Check sheet for the modelled part. Datum: model origin and axes. Units: mm. Face numbers are marked on the shaded views. A direction names the side the tool comes from. Give positions to 0.01 mm unless a question says otherwise; leave off trailing zeros. Order: outer loops, then holes, each group sorted by start corner. A loop starts at its lowest first (then second) coordinate and runs counter-clockwise, first axis right, second up. Notation, with made-up numbers: (61, 49) -> (119, 49) arc R18 cw to (119, 75) -> close; hole circle Ø5 at (-4.5, 14). An arc over 180 degrees is marked (long way). Write each question's results on one line, items separated by ' | '.
from build123d import *

# Parameters (mm, degrees)
F0_W     = 60
F0_H     = 30
F1_DEPTH = 5
F2_R     = 2.5
F3_DEPTH = 20
F4_R     = 0.75
F5_DEPTH = 23


with BuildPart() as f1:
    # F0 (on Top) → F1 (new body)
    with BuildSketch(Plane.XY):
        with Locations((6.484929, -2.445796)):
            Rectangle(F0_W, F0_H)
    extrude(amount=F1_DEPTH)

    # F2 (on face) → F3 (join)
    with BuildSketch(Plane.XY.offset(5)):
        with Locations((-16.015071, 5.054204)):
            Circle(F2_R)
        with Locations((-16.015071, -9.945796)):
            Circle(F2_R)
        with Locations((27.984929, 5.054204)):
            Circle(F2_R)
        with Locations((27.984929, -9.945796)):
            Circle(F2_R)
    extrude(amount=F3_DEPTH)

    # F4 (on face) → F5 (join)
    with BuildSketch(Plane.XY.offset(5)):
        with Locations((-16.015071, 5.054204)):
            Circle(F4_R)
        with Locations((-16.015071, -9.945796)):
            Circle(F4_R)
        with Locations((27.984929, 5.054204)):
            Circle(F4_R)
        with Locations((27.984929, -9.945796)):
            Circle(F4_R)
    extrude(amount=F5_DEPTH)


solid = f1.part
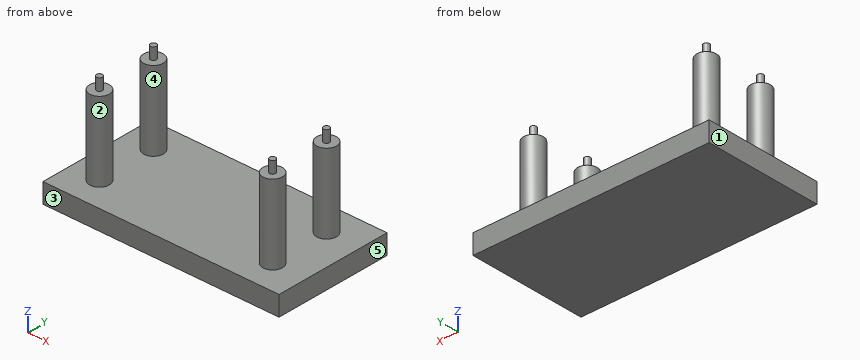
1. Gauge pin test, flat end, axial feed: pin 1 Ø8 at (x, y) = (1, -3.5) entering from +Z. Record the tip position at first contact, or that the pin passes through.
Verdict:
pin 1: stops at z = 5
2. Access from +Z, -Z, +X, -X, +Y, -Y to the whole of each face (thin tool, end or side, straight path). Record for the marked faces 1 and 2.
Verdict:
face 1: +Z, -Z, -X, +Y, -Y | face 2: +Z
3. Section check A-A on x = 9.5. Record the cut outline in (y, z).
Verdict:
outline: (-17.45, 0) -> (12.55, 0) -> (12.55, 5) -> (-17.45, 5) -> close
4. Section check B-B on y = 8.5. Record the cut outline in (x, z), then the cut area to 3 significant figures.
Verdict:
outline: (-23.52, 0) -> (36.48, 0) -> (36.48, 5) -> (-23.52, 5) -> close | area: 300 mm^2
5. Material ranges on probe 1 along X at (y, z) = (5.25, 8.5); probe 2 along Y at (x, z) = (-16, 18.75); probe 3 along Z at (x, y) = (25, -0.25), recorded low to high. Write a range as from..to.
Verdict:
probe 1: x = -18.51..-13.52, 25.49..30.48 | probe 2: y = -12.45..-7.45, 2.55..7.55 | probe 3: z = 0..5
6. Section check C-C on z = 7.5. Record the cut outline in (x, y).
Verdict:
outline: circle Ø5 at (-16.02, -9.95); circle Ø5 at (-16.02, 5.05); circle Ø5 at (27.98, -9.95); circle Ø5 at (27.98, 5.05)
7. Mould release check, pull along Y, two halves, no side actions. Record for the marked faces 3, 4 and 5: +Y half, -Y half, draft (parallel to the pull), parting line (faces both ways), or undercut.
Verdict:
face 3: -Y half | face 4: undercut | face 5: draft
